For this review, take the finished solid that the model builds, in its own axes (mm). A direction names the side the tool comes from. Give positions to 0.01 mm unless a question says otherwise; leave off trailing zeros. Write each loop counter-clockwise with the first axis right and the second up, starting at its lowest first coordinate (ties: lowest second). Pieces come first, ordered by that corner, then holes.
1) We need section A-A on z = -26. Give the boundary of the cut face in (x, y).
2) We need section B-B on x = -11. Give the boundary of the cut face in (y, z), and give its area (3 significant figures).
3) Machinability: for faces 1 (the face through (-23, 21, -9)), 2 (the face through (-12, -5.1, 7)), 3 (the face through (-14, 25.5, -5)), 4 (the face through (-11.878, 3.954, -49.821)), which of the approach directions +Z, -Z, +X, -X, +Y, -Y give a long, thin tool a straight path to every point of the face, cutting with its end or side? Answer none if there is none.
4) Wall thickness on line 1 along X through (y, z) = (-2.5, -13); line 2 along X through (y, z) = (3, -96.5); line 3 along Y through (x, z) = (7.5, -90): over which ranges is each line inside the solid? List them lowest first.
5) We need section C-C on x = 1. Give the boundary of the cut face in (y, z), and give its area (3 significant figures).
6) Draft analysis for pull direction Z (two halves, no side actions). For faces 5 (the face through (-11, 2, -99)), 6 (the face through (-10.08, 4.15, -57.52)), 7 (the face through (-24, 16, -4)), state which applies: pulls with the +Z half, pulls with the -Z half, needs draft (parallel to the pull), parting line crosses it, or undercut.
7) For P1, Ø1, axis at x = -2.5, y = 17.5, coming from the +Z side; P2, Ø9, axis at x = -15, y = 20, coming from the -Z side; P3, Ø2, axis at x = 2, z = -63, coming from the +Y side, all flat-tipped, find the tip position at first contact; note any pin that passes through.
8) We need section D-D on y = 15.5. Give the boundary of the cut face in (x, z), and give its area (3 significant figures).
from build123d import *

# Parameters (mm, degrees)
BOSS_EXTRUDE1_DEPTH      = 1
BOSS_EXTRUDE1_DEPTH_BACK = 112
SKETCH1_W                = 40
SKETCH1_H                = 12
SKETCH1_R                = 4.25
SKETCH3_R                = 2.55
BOSS_EXTRUDE2_DEPTH      = 15
CUT_EXTRUDE1_START       = -2.9
SKETCH3_2_R              = 2.55
CUT_EXTRUDE1_DEPTH       = 6.2
BOSS_EXTRUDE3_START      = -3
SKETCH5_R                = 4.25
BOSS_EXTRUDE3_DEPTH      = 3
CHAMFER3_SIZE            = 0.5
FILLET3_R                = 2
SKETCH12_R               = 4.05
BOSS_EXTRUDE9_DEPTH      = 100
SKETCH18_W               = 48
SKETCH18_H               = 21
BOSS_EXTRUDE11_DEPTH     = 10
FILLET10_R               = 2
CUT_EXTRUDE8_DEPTH       = 9
BOSS_EXTRUDE12_DEPTH     = 13


with BuildPart() as part:
    # Sketch1 → Boss-Extrude1 (new, two sides: drawn at the far end of the back side and taken through both)
    with BuildSketch(Plane.XY.offset(-BOSS_EXTRUDE1_DEPTH_BACK)):
        Rectangle(SKETCH1_W, SKETCH1_H)
        with Locations((11, 0)):
            Circle(SKETCH1_R, mode=Mode.SUBTRACT)
        with Locations(Location((-11, 0, 0), (0, 0, 180))):
            Circle(SKETCH1_R, mode=Mode.SUBTRACT)
    extrude(amount=BOSS_EXTRUDE1_DEPTH + BOSS_EXTRUDE1_DEPTH_BACK)

    # Sketch3 → Boss-Extrude2 (add, symmetric)
    with BuildSketch(Plane(origin=(0, 0, 0), x_dir=(0, 0, -1), z_dir=(1, 0, 0))):
        with BuildLine():
            Line((-12, -5.1), (-1, -5.1))
            Line((-1, -5.1), (-1, 5.1))
            Line((-1, 5.1), (-12, 5.1))
            ThreePointArc((-12, 5.1), (-17.1, 0), (-12, -5.1))
        make_face()
        with Locations((-12, 0)):
            Circle(SKETCH3_R, mode=Mode.SUBTRACT)
    extrude(amount=BOSS_EXTRUDE2_DEPTH, both=True)

    # Sketch3<2> → Cut-Extrude1 (cut)
    with BuildSketch(Plane(origin=(0, 0, 0), x_dir=(0, 0, -1), z_dir=(1, 0, 0)).offset(CUT_EXTRUDE1_START)):
        with BuildLine():
            Line((-12, -5.1), (-1, -5.1))
            Line((-1, -5.1), (-1, 5.1))
            Line((-1, 5.1), (-12, 5.1))
            ThreePointArc((-12, 5.1), (-17.1, 0), (-12, -5.1))
        make_face()
        with Locations((-12, 0)):
            Circle(SKETCH3_2_R, mode=Mode.SUBTRACT)
    cut_extrude1 = extrude(amount=-CUT_EXTRUDE1_DEPTH, mode=Mode.SUBTRACT)

    # Mirror1: Cut-Extrude1 across plane
    add(cut_extrude1.mirror(Plane(origin=(0, 0, 0), x_dir=(0, 0, 1), z_dir=(1, 0, 0))), mode=Mode.SUBTRACT)

    # Sketch5 → Boss-Extrude3 (add)
    with BuildSketch(Plane.XY.offset(1).offset(BOSS_EXTRUDE3_START)):
        with Locations((-11, 0)):
            Circle(SKETCH5_R)
        with Locations((11, 0)):
            Circle(SKETCH5_R)
    extrude(amount=BOSS_EXTRUDE3_DEPTH)

    # Chamfer3
    chamfer3_edges = [part.edges().sort_by_distance(p)[0] for p in [
        (6.75, 0, -112),
        (-20, 0, -112),
        (-6.75, 0, -112),
        (0, -6, -112),
        (20, 0, -112),
        (0, 6, -112),
    ]]
    chamfer(chamfer3_edges, length=CHAMFER3_SIZE)

    # Fillet3
    # the kernel refuses this fillet: 2 mm, written as the material it adds along each edge
    with BuildSketch(Plane(origin=(9.1, -5.1, 1), x_dir=(0, -1.0, 1.5367953823073576e-12), z_dir=(1, 0, 0)), Plane(origin=(-15, -5.1, 1), x_dir=(0, -1.0, 1.5367953823073576e-12), z_dir=(1, 0, 0))) as fillet3_piece_1:
        with BuildLine():
            CenterArc((2, -1.670329309), FILLET3_R, 123.367012969, 56.632987031)
            Line((0, -1.670329309), (-0.04, -1.670329309))
            Line((-0.04, -1.670329309), (-0.04, 0))
            Line((-0.04, 0), (0, 0.04))
            ThreePointArc((0, 0.04), (0.45, 0.04), (0.878, 0.033406586))
            Line((0.878, 0.033406586), (0.9, 0))
        make_face()
    extrude(amount=5.9)
    with BuildSketch(Plane(origin=(9.1, 5.1, 1), x_dir=(0, 1.0, 1.5343282200304168e-12), z_dir=(1, 0, 0)), Plane(origin=(-15, 5.1, 1), x_dir=(0, 1.0, 1.5340815038027225e-12), z_dir=(1, 0, 0))) as fillet3_piece_2:
        with BuildLine():
            CenterArc((2, 1.670329309), FILLET3_R, 180, 56.632987031)
            Line((0, 1.670329309), (-0.04, 1.670329309))
            Line((-0.04, 1.670329309), (-0.04, 0))
            Line((-0.04, 0), (0, -0.04))
            ThreePointArc((0, -0.04), (0.45, -0.04), (0.878, -0.033406586))
            Line((0.878, -0.033406586), (0.9, 0))
        make_face()
    extrude(amount=5.9)
    with BuildSketch(Plane(origin=(-2.9, 5.1, 1), x_dir=(0, 1.0, 1.5343282200304168e-12), z_dir=(1, 0, 0))) as fillet3_piece_3:
        with BuildLine():
            CenterArc((2, 1.670329309), FILLET3_R, 180, 56.632987031)
            Line((0, 1.670329309), (-0.04, 1.670329309))
            Line((-0.04, 1.670329309), (-0.04, 0))
            Line((-0.04, 0), (0, -0.04))
            ThreePointArc((0, -0.04), (0.45, -0.04), (0.878, -0.033406586))
            Line((0.878, -0.033406586), (0.9, 0))
        make_face()
    extrude(amount=5.8)
    with BuildSketch(Plane(origin=(-2.9, -5.1, 1), x_dir=(0, -1.0, 1.5367953823073576e-12), z_dir=(1, 0, 0))) as fillet3_piece_4:
        with BuildLine():
            CenterArc((2, -1.670329309), FILLET3_R, 123.367012969, 56.632987031)
            Line((0, -1.670329309), (-0.04, -1.670329309))
            Line((-0.04, -1.670329309), (-0.04, 0))
            Line((-0.04, 0), (0, 0.04))
            ThreePointArc((0, 0.04), (0.45, 0.04), (0.878, 0.033406586))
            Line((0.878, 0.033406586), (0.9, 0))
        make_face()
    extrude(amount=5.8)

    # Sketch12 → Boss-Extrude9 (add)
    with BuildSketch(Plane(origin=(0, 0, 1), x_dir=(-1, 0, 0), z_dir=(0, 0, -1))):
        with Locations(Location((11, 0, 0), (0, 0, 180))):
            Circle(SKETCH12_R)
        with Locations(Location((-11, 0, 0), (0, 0, 180))):
            Circle(SKETCH12_R)
    extrude(amount=BOSS_EXTRUDE9_DEPTH)

    # Sketch18 → Boss-Extrude11 (add)
    with BuildSketch(Plane(origin=(0, 0, 1), x_dir=(-1, 0, 0), z_dir=(0, 0, -1))):
        with Locations((0, 16.5)):
            Rectangle(SKETCH18_W, SKETCH18_H)
    extrude(amount=BOSS_EXTRUDE11_DEPTH)

    # Fillet10
    fillet10_edges = [part.edges().sort_by_distance(p)[0] for p in [
        (-24, 6, -4),
        (-24, 27, -4),
        (24, 27, -4),
        (24, 6, -4),
    ]]
    fillet(fillet10_edges, radius=FILLET10_R)

    # Sketch20 → Cut-Extrude8 (cut)
    with BuildSketch(Plane(origin=(0, 0, -9), x_dir=(-1, 0, 0), z_dir=(0, 0, -1))):
        with BuildLine():
            Line((-22.5, 24.5), (-22.5, 6))
            Line((-22.5, 6), (22.5, 6))
            Line((22.5, 6), (22.5, 24.5))
            ThreePointArc((22.5, 24.5), (22.207106781, 25.207106781), (21.5, 25.5))
            Line((21.5, 25.5), (5.5, 25.5))
            Line((5.5, 25.5), (5.5, 27))
            Line((5.5, 27), (-5.5, 27))
            Line((-5.5, 27), (-5.5, 25.5))
            Line((-5.5, 25.5), (-21.5, 25.5))
            ThreePointArc((-21.5, 25.5), (-22.207106781, 25.207106781), (-22.5, 24.5))
        make_face()
    extrude(amount=-CUT_EXTRUDE8_DEPTH, mode=Mode.SUBTRACT)

    # Sketch22 → Boss-Extrude12 (add)
    with BuildSketch(Plane(origin=(0, 0, -99), x_dir=(-1, 0, 0), z_dir=(0, 0, -1))):
        with BuildLine():
            Line((15.75, 0), (6.25, 0))
            ThreePointArc((6.25, 0), (11, -4.75), (15.75, 0))
        make_face()
        with BuildLine():
            Line((-6.25, 0), (-15.75, 0))
            ThreePointArc((-15.75, 0), (-11, -4.75), (-6.25, 0))
        make_face()
    extrude(amount=BOSS_EXTRUDE12_DEPTH)


solid = part.part
Results list:
1. outline: (-20, -6) - (20, -6) - (20, 6) - (-20, 6) - close; circle Ø8.1 at (-11, 0); circle Ø8.1 at (11, 0); hole circle Ø8.5 at (-11, 0); hole circle Ø8.5 at (11, 0)
2. outline: (-6, -111.5) - (-5.5, -112) - (0, -112) - (0, -99) - (4.05, -99) - (4.05, -2) - (4.25, -2) - (4.25, -111.5) - (4.75, -112) - (5.5, -112) - (6, -111.5) - (6, 0) - (25.5, 0) - (25.5, -9) - (27, -9) - (27, 1) - (6, 1) arc R2 cw to (5.1, 2.67) - (5.1, 12) arc R5.1 ccw to (-5.1, 12) - (-5.1, 2.67) arc R2 cw to (-6, 1) - close; hole (-4.25, -99) - (-4.05, -99) - (-4.05, -2) - (-4.25, -2) - close; hole circle Ø5.1 at (0, 12)
2. area: 1,430 mm2
3. face 1: -Z, +X, -X, +Y
3. face 2: +Z, +X, -X, -Y
3. face 3: -Z
3. face 4: none
4. line 1: x = -20 to -14.44, -14.19 to -7.81, -7.56 to 7.56, 7.81 to 14.19, 14.44 to 20
4. line 2: x = -20 to -14.01, -13.72 to -8.28, -7.99 to 7.99, 8.28 to 13.72, 14.01 to 20
4. line 3: y = -6 to -2.41, -2.04 to 2.04, 2.41 to 6
5. outline: (-6, -111.5) - (-5.5, -112) - (5.5, -112) - (6, -111.5) - (6, 0) - (27, 0) - (27, 1) - (6, 1) arc R2 cw to (5.1, 2.67) - (5.1, 12) arc R5.1 ccw to (-5.1, 12) - (-5.1, 2.67) arc R2 cw to (-6, 1) - close; hole circle Ø5.1 at (0, 12)
5. area: 1,510 mm2
6. face 5: pulls with the -Z half
6. face 6: undercut
6. face 7: needs draft
7. P1: stops at z = 1
7. P2: stops at z = 0
7. P3: stops at y = 6
8. outline: (-24, -9) - (-22.5, -9) - (-22.5, 0) - (22.5, 0) - (22.5, -9) - (24, -9) - (24, 1) - (-24, 1) - close
8. area: 75.0 mm2
